from build123d import *

# Parameters (mm, degrees)
SKETCH_R        = 14
SKETCH_R_2      = 1.25
PAD_DEPTH       = 2
SKETCH001_R     = 5
POCKET_DEPTH    = 1
SKETCH002_R     = 2.5
POCKET001_DEPTH = 1


with BuildPart() as part:
    # Sketch → Pad (new body)
    with BuildSketch(Plane.XY):
        Circle(SKETCH_R)
        with Locations((0, 11)):
            Circle(SKETCH_R_2, mode=Mode.SUBTRACT)
        with Locations((-11, 0)):
            Circle(SKETCH_R_2, mode=Mode.SUBTRACT)
        with Locations((0, -11)):
            Circle(SKETCH_R_2, mode=Mode.SUBTRACT)
        with Locations((11, 0)):
            Circle(SKETCH_R_2, mode=Mode.SUBTRACT)
    extrude(amount=PAD_DEPTH)

    # Sketch001 (on Face7 of Pad) → Pocket (cut)
    with BuildSketch(Plane.XY.offset(2)):
        Circle(SKETCH001_R)
    extrude(amount=-POCKET_DEPTH, mode=Mode.SUBTRACT)

    # Sketch002 (on Face2 of Pocket) → Pocket001 (cut)
    with BuildSketch(Plane(origin=(0, 0, 0), x_dir=(1, 0, 0), z_dir=(0, 0, -1))):
        with Locations((0, 11)):
            Circle(SKETCH002_R)
        with Locations((11, 0)):
            Circle(SKETCH002_R)
        with Locations((-11, 0)):
            Circle(SKETCH002_R)
        with Locations((0, -11)):
            Circle(SKETCH002_R)
    extrude(amount=-POCKET001_DEPTH, mode=Mode.SUBTRACT)


solid = part.part
Verification items for the finished model (mm, model axes). A direction names the side the tool comes from. Coordinates: 2 decimals unless noted, no trailing zeros. Write each loop counter-clockwise with the first axis right and the second up, starting at its lowest first coordinate (ties: lowest second). Pieces come first, ordered by that corner, then holes. Notation, with made-up numbers: M -26,69.5 L 23,69.5 A13 ccw 23,78.5 Z; hole C 5.25,65.25 d6. An arc over 180 degrees is marked long. Use CSV: the item, a comma, the result in double quotes.
Q1. Go/stop test with flat-tipped pins: P1, Ø3, axis at x = 0, y = -11, coming from the -Z side; P2, Ø8, axis at x = 0, y = 0, coming from the -Z side; P3, Ø3, axis at x = 0.5, y = 2, coming from the +Z side; P4, Ø2, axis at x = 11, y = 0, coming from the +Z side. Record where each tip stops, or that it passes through.
Computed values:
P1,"z = 1"
P2,"z = 0"
P3,"z = 1"
P4,"through"
Q2. Section check A-A, the plane y = 0. Enter the section's corners in (x, z).
Computed values:
outline,"M -14,0 L -13.5,0 L -13.5,1 L -12.25,1 L -12.25,2 L -14,2 Z; M -9.75,1 L -8.5,1 L -8.5,0 L 8.5,0 L 8.5,1 L 9.75,1 L 9.75,2 L 5,2 L 5,1 L -5,1 L -5,2 L -9.75,2 Z; M 12.25,1 L 13.5,1 L 13.5,0 L 14,0 L 14,2 L 12.25,2 Z"
Q3. Thickness scan on line 1 along Y through (x, z) = (0, 1.75); line 2 along Y through (x, z) = (0, 0.3); line 3 along X through (y, z) = (-0.5, 0.4). Record the ranges inside material, lowest first. Write a range as [from, to].
Computed values:
line 1,"[-14, -12.25], [-9.75, -5], [5, 9.75], [12.25, 14]"
line 2,"[-14, -13.5], [-8.5, 8.5], [13.5, 14]"
line 3,"[-13.99, -13.45], [-8.55, 8.55], [13.45, 13.99]"
Q4. Section check D-D, the plane y = 11. Enter the section's corners in (x, z), and give its area (3 significant figures).
Computed values:
outline,"M -8.66,0 L -2.5,0 L -2.5,1 L -1.25,1 L -1.25,2 L -8.66,2 Z; M 1.25,1 L 2.5,1 L 2.5,0 L 8.66,0 L 8.66,2 L 1.25,2 Z"
area,"27.1 mm²"
Q5. Set-up check for faces 1 (the cylindrical face through (-1.08, -4.88, 1.51)), 2 (the flat face through (0, 0, 0)), 3 (the flat face through (-1, -10, 1)): record each of +Z, -Z, +X, -X, +Y, -Y from which the full face is reachable in a straight line by a thin tool's end or side.
Computed values:
face 1,"+Z"
face 2,"-Z, +X, -X, +Y, -Y"
face 3,"-Z"
Q6. Mould release check, pull along X, two halves, no side actions. Record for faces 4 (the flat face through (0, 0, 1)), 5 (the flat face through (0, -6, 2)), 6 (the cylindrical face through (-0.16, -9.76, 1.49)), 7 (the cylindrical face through (12.932, -5.362, 0.986)): pulls with the +X half, pulls with the -X half, needs draft (parallel to the pull), parting line crosses it, or undercut.
Computed values:
face 4,"undercut"
face 5,"needs draft"
face 6,"undercut"
face 7,"parting line crosses it"
Q7. Section check C-C, the plane z = 0.55. Enter the section's corners in (x, y).
Computed values:
outline,"C 0,0 d28; hole C -11,0 d5; hole C 0,-11 d5; hole C 0,11 d5; hole C 11,0 d5"
